Input: part model. Units: mm. Frame: model coordinates. Face numbers are marked on the shaded views. A direction names the side the tool comes from. Coordinates: 2 decimals unless noted, no trailing zeros. Order: outer loops, then holes, each group sorted by start corner. A loop starts at its lowest first (then second) coordinate and runs counter-clockwise, first axis right, second up. Notation, with made-up numbers: (-11.5, -36) -> (22.5, -36) arc R30 ccw to (22.5, -5) -> close; hole circle Ø3 at (-4.75, 30.25). An arc over 180 degrees is marked (long way). Write each question's results on one line, items separated by ' | '.
```python
from build123d import *

# Parameters (mm, degrees)
SKETCH1_R               = 0.5
SKETCH1_R_2             = 1
BOSS_EXTRUDE1_DEPTH     = 1.5
CUT_EXTRUDE1_DEPTH      = 11.41549897
CUT_EXTRUDE1_DEPTH_BACK = 1
FILLET1_R               = 0.8


with BuildPart() as part:
    # Sketch1 → Boss-Extrude1 (new body)
    with BuildSketch(Plane.XY):
        with BuildLine():
            Line((6, -27.5), (1.693454448, -46.525168442))
            ThreePointArc((1.693454448, -46.525168442), (2.428871416, -50.096858061), (5.6, -51.897343647))
            Line((5.6, -51.897343647), (5.6, -74.316095527))
            Line((5.6, -74.316095527), (6.4, -74.316095527))
            Line((6.4, -74.316095527), (6.4, -51.897343647))
            ThreePointArc((6.4, -51.897343647), (9.571128584, -50.096858061), (10.306545552, -46.525168442))
            Line((10.306545552, -46.525168442), (6, -27.5))
        make_face()
        with Locations((6, -33)):
            Circle(SKETCH1_R, mode=Mode.SUBTRACT)
        with Locations((6, -45)):
            Circle(SKETCH1_R_2, mode=Mode.SUBTRACT)
    extrude(amount=BOSS_EXTRUDE1_DEPTH)

    # Sketch2 → Cut-Extrude1 (cut, two sides)
    with BuildSketch(Plane(origin=(0, 0, 0), x_dir=(0, 0, -1), z_dir=(1, 0, 0))) as cut_extrude1_sk:
        with BuildLine():
            Line((-1.5, -14.744083324), (-0.5, -14.744083324))
            Line((-0.5, -14.744083324), (-0.5, -46.897343647))
            ThreePointArc((-0.5, -46.897343647), (-0.792893219, -47.604450429), (-1.5, -47.897343647))
            Line((-1.5, -47.897343647), (-1.5, -14.744083324))
        make_face()
    extrude(amount=CUT_EXTRUDE1_DEPTH, mode=Mode.SUBTRACT)
    extrude(cut_extrude1_sk.sketch, amount=-CUT_EXTRUDE1_DEPTH_BACK, mode=Mode.SUBTRACT)

    # Fillet1
    fillet1_edges = [part.edges().sort_by_distance(p)[0] for p in [
        (6, -27.5, 0.25),
    ]]
    fillet(fillet1_edges, radius=FILLET1_R)


solid = part.part
```
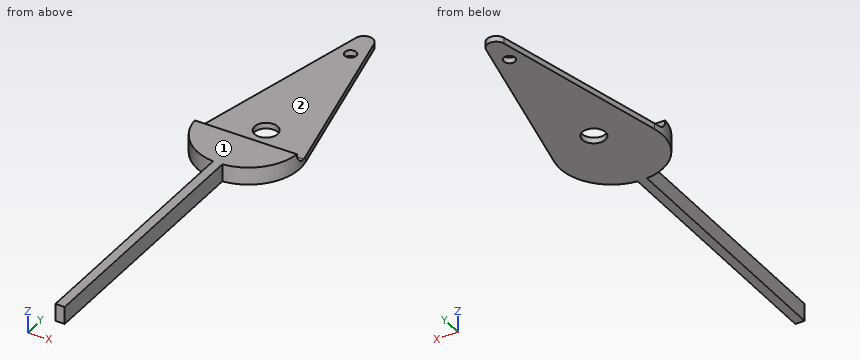
(1) Cut plane B-B, the plane y = -33. Return loops of the section in (x, z), plus the area to 3 significant figures.
Return value:
outline: (4.76, 0) -> (5.5, 0) -> (5.5, 0.5) -> (4.76, 0.5) -> close; (6.5, 0) -> (7.24, 0) -> (7.24, 0.5) -> (6.5, 0.5) -> close | area: 0.745 mm2
(2) Reachability of the marked faces 1 and 2 from +Z, -Z, +X, -X, +Y, -Y: full face, straight path, thin tool, end or side. Return the list, or none.
Return value:
face 1: +Z, +X, -X, +Y, -Y | face 2: +Z, +X, -X, +Y
(3) Line query: line 1 along Y through (x, z) = (6, 0.35); line 2 along Z through (x, y) = (7.5, -40); line 3 along X through (y, z) = (-58, 0.2). Output: solid intervals per line, ascending. Write a range as from..to.
Return value:
line 1: -74.32..-46, -44..-33.5, -32.5..-30.32 | line 2: 0..0.5 | line 3: 5.6..6.4
(4) Cut plane C-C, the plane z = 1. Return loops of the section in (x, y).
Return value:
outline: (1.59, -47.76) arc R4.42 ccw to (5.6, -51.9) -> (5.6, -74.32) -> (6.4, -74.32) -> (6.4, -51.9) arc R4.42 ccw to (10.41, -47.76) -> close
(5) Cut plane A-A, the plane x = 6. Return loops of the section in (y, z), plus the area to 3 significant figures.
Return value:
outline: (-74.32, 0) -> (-46, 0) -> (-46, 0.5) -> (-46.9, 0.5) arc R1 cw to (-47.9, 1.5) -> (-74.32, 1.5) -> close; (-44, 0) -> (-33.5, 0) -> (-33.5, 0.5) -> (-44, 0.5) -> close; (-32.5, 0) -> (-30.32, 0) -> (-30.32, 0.5) -> (-32.5, 0.5) -> close | area: 47.1 mm2
(6) Pin query (flat end, axial travel): P1, Ø5, axis at x = 3, y = -63.5, coming from the -Z side; P2, Ø0.8, axis at y = -62, z = 0.5, coming from the +X side. Return the tip coordinate at first contact, or that it passes through.
Return value:
P1: through | P2: x = 6.4
(7) Cut plane D-D, the plane y = -60.5. Return loops of the section in (x, z).
Return value:
outline: (5.6, 0) -> (6.4, 0) -> (6.4, 1.5) -> (5.6, 1.5) -> close
